Source: CAD feature listing. Evaluate the final solid. Frame: model axes, mm. A direction names the side the tool comes from. Coordinates: 2 decimals unless noted, no trailing zeros. Order: outer loops, then holes, each group sorted by start corner. A loop starts at its lowest first (then second) coordinate and runs counter-clockwise, first axis right, second up.
Item 1: Ray query, line 1 (X direction, y = 14, z = 1.3); line 2 (X direction, y = 5, z = 3.6); line 3 (Y direction, x = -114.5, z = 1.4). Return the intervals inside material, ascending.
Item 2: Reachability of faces 1 (the flat face through (-140.792, 0, 2)), 2 (the flat face through (-48, 1, 5)), 3 (the flat face through (0, -31.8, 3)), 4 (the flat face through (-102, -10, 2)), 5 (the flat face through (-103, 10, 2)) from +Z, -Z, +X, -X, +Y, -Y: full face, straight path, thin tool, end or side. Return the list, or none.
Item 3: Section A-A on x = 0. Return the cut outline in (y, z).
Item 4: Section D-D on x = -57.5. Return the cut outline in (y, z).
Item 5: Contact query for flat-ended pins moving along their axis: P1, Ø1.5, axis at x = -99, z = 3, coming from the +Y side; P2, Ø1.5, axis at x = -6, z = 4, coming from the +Y side; P3, Ø1.7, axis at x = 0.5, z = 3, coming from the +Y side. Output: stop coordinate, or through.
Item 6: Section C-C on x = -112. Return the cut outline in (y, z), then the cut area to 3 significant figures.
Item 7: Mould query, pull axis X, two halves, no side actions, for faces 6 (the cylindrical face through (-21.27, -21.156, 2.535)), 7 (the flat face through (-48, 1, 0)), 8 (the cylindrical face through (41.975, -1.461, 2.465)). Classes: released by +X, released by -X, zero draft, split by the parting line, or undercut.
Item 8: Section B-B on y = 0. Return the cut outline in (x, z), then the cut area to 3 significant figures.
from build123d import *

# Parameters (mm, degrees)
PAD_DEPTH          = 5
SKETCH001_R        = 30
POCKET_DEPTH       = 5.001
POCKET001_DEPTH    = 407.463283
POLARPATTERN_COUNT = 12
FILLET_R           = 40
FILLET001_R        = 40


with BuildPart() as part:
    # Sketch → Pad (new body)
    with BuildSketch(Plane.XY):
        with BuildLine():
            Line((-140.792156, 10), (-40.792156, 10))
            ThreePointArc((-40.792156, -10), (42, 0), (-40.792156, 10))
            Line((-40.792156, -10), (-140.792156, -10))
            Line((-140.792156, -10), (-140.792156, 10))
        make_face()
    extrude(amount=PAD_DEPTH)

    # Sketch001 → Pocket (cut, through all)
    with BuildSketch(Plane.XY.offset(5)):
        Circle(SKETCH001_R)
    extrude(amount=-POCKET_DEPTH, mode=Mode.SUBTRACT)

    # Sketch002 → Pocket001 (cut, through all)
    with BuildSketch(Plane.XY.offset(5)):
        Polygon((-1.65, 31.8), (-2.15, 29.8), (2.15, 29.8), (1.65, 31.8), align=None)
    pocket001 = extrude(amount=-POCKET001_DEPTH, mode=Mode.SUBTRACT)

    # PolarPattern: Pocket001 ×12 about axis
    polarpattern_axis = Axis((0, 0, 5), (0, 0, 1))
    for i in range(1, POLARPATTERN_COUNT):
        add(pocket001.rotate(polarpattern_axis, i * 360 / POLARPATTERN_COUNT), mode=Mode.SUBTRACT)

    # Fillet
    fillet_edges = [part.edges().sort_by_distance(p)[0] for p in [
        (-40.792156, -10, 2.5),
    ]]
    fillet(fillet_edges, radius=FILLET_R)

    # Fillet001
    fillet001_edges = [part.edges().sort_by_distance(p)[0] for p in [
        (-40.792156, 10, 2.5),
    ]]
    fillet(fillet001_edges, radius=FILLET001_R)


solid = part.part
Answer list:
1. line 1: x = -47.56 to -27.88, 27.88 to 39.6
1. line 2: x = -140.79 to -29.58, 29.58 to 41.7
1. line 3: y = -10 to 10
2. face 1: +Z, -Z, -X, +Y, -Y
2. face 2: +Z, +X, -X, +Y, -Y
2. face 3: +Z, -Z
2. face 4: +Z, -Z, -X, -Y
2. face 5: +Z, -Z, -X, +Y
3. outline: (-42, 0) - (-31.8, 0) - (-31.8, 5) - (-42, 5) - close; (31.8, 0) - (42, 0) - (42, 5) - (31.8, 5) - close
4. outline: (-10.71, 0) - (10.71, 0) - (10.71, 5) - (-10.71, 5) - close
5. P1: stops at y = 10
5. P2: stops at y = 41.67
5. P3: stops at y = 42
6. outline: (-10, 0) - (10, 0) - (10, 5) - (-10, 5) - close
6. area: 100 mm2
7. face 6: undercut
7. face 7: zero draft
7. face 8: split by the parting line
8. outline: (-140.79, 0) - (-31.8, 0) - (-31.8, 5) - (-140.79, 5) - close; (31.8, 0) - (42, 0) - (42, 5) - (31.8, 5) - close
8. area: 596 mm2
